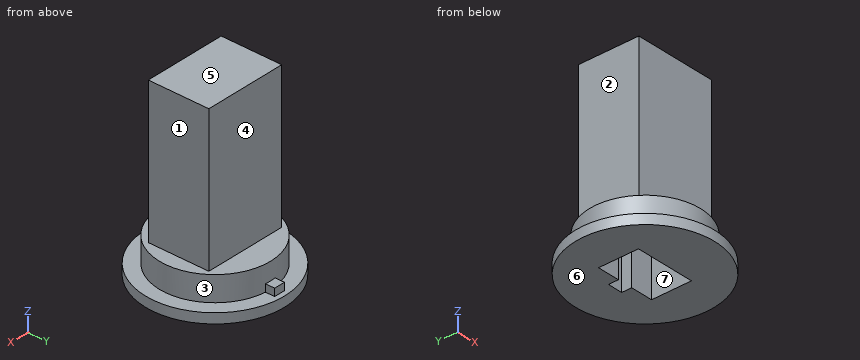
```python
from build123d import *

# Parameters (mm, degrees)
ESQUISSE1_R             = 13.95
BOSS_EXTRU_1_DEPTH      = 2
ESQUISSE2_R             = 11.15
BOSS_EXTRU_2_DEPTH      = 5
BOSS_EXTRU_3_DEPTH      = 1.5
ESQUISSE4_W             = 16.5
ESQUISSE4_H             = 12.15
BOSS_EXTRU_4_DEPTH      = 28.9
ENL_V_MAT_EXTRU_1_DEPTH = 10


with BuildPart() as part:
    # Esquisse1 → Boss.-Extru.1 (new body)
    with BuildSketch(Plane.XY):
        Circle(ESQUISSE1_R)
    extrude(amount=BOSS_EXTRU_1_DEPTH)

    # Esquisse2 → Boss.-Extru.2 (add)
    with BuildSketch(Plane.XY.offset(2)):
        Circle(ESQUISSE2_R)
    extrude(amount=BOSS_EXTRU_2_DEPTH)

    # Esquisse3 → Boss.-Extru.3 (add)
    with BuildSketch(Plane.XY.offset(2)):
        with BuildLine():
            ThreePointArc((-1.1, 11.095607239), (0, 11.15), (1.1, 11.095607239))
            Line((1.1, 11.095607239), (1.1, 12.95))
            Line((1.1, 12.95), (-1.1, 12.95))
            Line((-1.1, 12.95), (-1.1, 11.095607239))
        make_face()
    extrude(amount=BOSS_EXTRU_3_DEPTH)

    # Esquisse4 → Boss.-Extru.4 (add)
    with BuildSketch(Plane.XY.offset(7)):
        Rectangle(ESQUISSE4_W, ESQUISSE4_H)
    extrude(amount=BOSS_EXTRU_4_DEPTH)

    # Esquisse6 → Enlèv. mat.-Extru.1 (cut)
    with BuildSketch(Plane(origin=(0, 0, 0), x_dir=(-1, 0, 0), z_dir=(0, 0, -1))):
        Polygon((6, 4), (1.5, 4), (1.5, 6), (-1.5, 6), (-1.5, 4), (-6, 4), (-6, -4), (6, -4), align=None)
    extrude(amount=-ENL_V_MAT_EXTRU_1_DEPTH, mode=Mode.SUBTRACT)


solid = part.part
```
Input: part model. Units: mm. Frame: model coordinates. Face numbers are marked on the shaded views. A direction names the side the tool comes from. Give positions to 0.01 mm unless a question says otherwise; leave off trailing zeros. Order: outer loops, then holes, each group sorted by start corner. A loop starts at its lowest first (then second) coordinate and runs counter-clockwise, first axis right, second up.
1. Mould query, pull axis Z, two halves, no side actions, for the marked faces 5, 6 and 7. Classes: released by +Z, released by -Z, zero draft, split by the parting line, or undercut.
Derived:
face 5: released by +Z
face 6: released by -Z
face 7: zero draft
2. Section C-C on z = 23.5. Return the cut outline in (x, y) (3 decimals), and give its area (3 significant figures).
Derived:
outline: (-8.25, -6.075) - (8.25, -6.075) - (8.25, 6.075) - (-8.25, 6.075) - close
area: 200 mm2
3. Reachability of the marked faces 1, 2, 3 and 4 from +Z, -Z, +X, -X, +Y, -Y: full face, straight path, thin tool, end or side. Return the list, or none.
Derived:
face 1: +Z, +X, +Y, -Y
face 2: +Z, -X, +Y, -Y
face 3: +Z
face 4: +Z, +X, -X, +Y
4. Section A-A on y = 0. Return the cut outline in (x, z).
Derived:
outline: (-13.95, 0) - (-6, 0) - (-6, 10) - (6, 10) - (6, 0) - (13.95, 0) - (13.95, 2) - (11.15, 2) - (11.15, 7) - (8.25, 7) - (8.25, 35.9) - (-8.25, 35.9) - (-8.25, 7) - (-11.15, 7) - (-11.15, 2) - (-13.95, 2) - close
5. Material intervals for L1, parallel to Y at x = -4.5, z = 23 (3 decimals); L2, parallel to X at y = 3.25, z = 31.5; L3, parallel to Z at x = -2.25, y = 10.5, sorted ascending.
Derived:
L1: y = -6.075 to 6.075
L2: x = -8.25 to 8.25
L3: z = 0 to 7
6. Section D-D on y = -3.5. Return the cut outline in (x, z).
Derived:
outline: (-13.5, 0) - (-6, 0) - (-6, 10) - (6, 10) - (6, 0) - (13.5, 0) - (13.5, 2) - (10.59, 2) - (10.59, 7) - (8.25, 7) - (8.25, 35.9) - (-8.25, 35.9) - (-8.25, 7) - (-10.59, 7) - (-10.59, 2) - (-13.5, 2) - close
7. Pin query (flat end, axial travel): pin 1 (2 mm diameter, centred on y = -4.5, z = 21, fed in from -X); pin 2 (1 mm diameter, centred on x = -6, z = 6.5, fed in from -Y); pin 3 (0.9 mm diameter, centred on x = -0.5, y = 11.5, fed in from +Z). Return the tip coordinate at first contact, or that it passes through.
Derived:
pin 1: stops at x = -8.25
pin 2: stops at y = -9.7
pin 3: stops at z = 7
8. Section B-B on x = 0. Return the cut outline in (y, z) (3 decimals), and give its area (3 significant figures).
Derived:
outline: (-13.95, 0) - (-4, 0) - (-4, 10) - (6, 10) - (6, 0) - (13.95, 0) - (13.95, 2) - (12.95, 2) - (12.95, 3.5) - (11.15, 3.5) - (11.15, 7) - (6.075, 7) - (6.075, 35.9) - (-6.075, 35.9) - (-6.075, 7) - (-11.15, 7) - (-11.15, 2) - (-13.95, 2) - close
area: 421 mm2
